from build123d import *

# Parameters (mm, degrees)
SM_BASE_FLANGE_1_DEPTH = 5
OTHER_START            = -15
OTHER_1_OUTLINE_W      = 5
OTHER_1_OUTLINE_H      = 5
OTHER_1_DEPTH          = 27


# Read off the part's stored shape, not the designer's step: Полость1
# Sheet-metal steps are written as plain solids
with BuildPart() as part:
    # Sketch 1 → Базовая кромка1 (new body)
    with BuildSketch(Plane(origin=(0, 0, 0), x_dir=(1, 0, 0), z_dir=(0, 1, 0))):
        Polygon((-15, 0), (-15, 92), (15, 92), (56, 0), align=None)
    extrude(amount=SM_BASE_FLANGE_1_DEPTH)

    # Полость1 outline → Полость1 (cut)
    with BuildSketch(Plane.YZ.offset(OTHER_START)):
        with Locations((2.5, -13)):
            Rectangle(OTHER_1_OUTLINE_W, OTHER_1_OUTLINE_H)
    extrude(amount=OTHER_1_DEPTH, mode=Mode.SUBTRACT)


solid = part.part
Geometry: final body of the model. Coordinates: model frame, mm. A direction names the side the tool comes from. Give positions to 0.01 mm unless a question says otherwise; leave off trailing zeros. Write each loop counter-clockwise with the first axis right and the second up, starting at its lowest first coordinate (ties: lowest second). Pieces come first, ordered by that corner, then holes. Notation, with made-up numbers: M 33,32 L 84,32 A23 ccw 84,62 Z; hole C 76.25,-33 d3. An arc over 180 degrees is marked long. Answer in a Markdown table with one row per item. Add a question column.
(1) Section B-B on y = 3.5. Return loops of the section in (x, z).
(2) Ray query, line 1 (Z direction, x = 8, y = 4.6); line 2 (X direction, y = 2.1, z = -80.5) (3 decimals); line 3 (Z direction, x = 38.5, y = 0.95). Return the intervals inside material, ascending.
(3) Section A-A on x = 9. Return loops of the section in (y, z), and give its area (3 significant figures).
(4) Reachability of faces 1 (the flat face through (-2, 2, -10.5)), 2 (the flat face through (13, 5, -36)) from +Z, -Z, +X, -X, +Y, -Y: full face, straight path, thin tool, end or side. Return the list, or none.
(5) Section C-C on x = 35.5. Return loops of the section in (y, z).
(6) Section D-D on z = -22.5. Return loops of the section in (x, y).
(7) First-contact query: pin 1 (1.5 mm diameter, centred on y = 3, z = -13, fed in from -X). Flat tip, straight axial feed; report the tip coordinate or a pass-through.
(8) Mould query, pull axis Z, two halves, no side actions, for faces 3 (the flat face through (13, 0, -36)), 4 (the flat face through (-2, 2, -15.5)), 5 (the flat face through (0, 2, -92)), 6 (the flat face through (12, 2, -13)). Classes: +Z half, -Z half, draft (parallel to the pull), parting line (faces both ways), or undercut.
Result set:
| question | item | result |
|---|---|---|
| 1 | outline | M -15,-92 L 15,-92 L 56,0 L -15,0 L -15,-10.5 L 12,-10.5 L 12,-15.5 L -15,-15.5 Z |
| 2 | line 1 | z = -92 to -15.5, -10.5 to 0 |
| 2 | line 2 | x = -15 to 20.125 |
| 2 | line 3 | z = -39.27 to 0 |
| 3 | outline | M 0,-92 L 5,-92 L 5,-15.5 L 0,-15.5 Z; M 0,-10.5 L 5,-10.5 L 5,0 L 0,0 Z |
| 3 | area | 435 mm^2 |
| 4 | face 1 | -X, +Y, -Y |
| 4 | face 2 | +Z, -Z, +X, -X, +Y |
| 5 | outline | M 0,-46 L 5,-46 L 5,0 L 0,0 Z |
| 6 | outline | M -15,0 L 45.97,0 L 45.97,5 L -15,5 Z |
| 7 | pin 1 | stops at x = 12 |
| 8 | face 3 | draft |
| 8 | face 4 | undercut |
| 8 | face 5 | -Z half |
| 8 | face 6 | undercut |
